from build123d import *
from build123d.topology import SkipClean

# Parameters (mm, degrees)
SALIENTE_EXTRUIR1_DEPTH    = 2.4
CORTAR_EXTRUIR1_DEPTH      = 15.629080627
CORTAR_EXTRUIR1_DEPTH_BACK = 15.629080627
CROQUIS2_R                 = 1.5
CROQUIS3_R                 = 1.5
SALIENTE_EXTRUIR2_DEPTH    = 7.5
CORTAR_EXTRUIR2_DEPTH      = 3.1
REDONDEO1_R                = 2
REDONDEO2_R                = 1


with BuildPart() as part:
    # Croquis1 → Saliente-Extruir1 (new, symmetric)
    with BuildSketch(Plane(origin=(0, 0, 0), x_dir=(0, 0, -1), z_dir=(1, 0, 0))):
        with BuildLine():
            Line((-13, 3.5), (13, 3.5))
            ThreePointArc((13, 3.5), (13.707106781, 3.207106781), (14, 2.5))
            Line((14, 2.5), (14, -2.5))
            Line((14, -2.5), (14, -3.5))
            Line((14, -3.5), (13, -3.5))
            Line((13, -3.5), (-13, -3.5))
            ThreePointArc((-13, -3.5), (-13.707106781, -3.207106781), (-14, -2.5))
            Line((-14, -2.5), (-14, 2.5))
            ThreePointArc((-14, 2.5), (-13.707106781, 3.207106781), (-13, 3.5))
        make_face()
    extrude(amount=SALIENTE_EXTRUIR1_DEPTH, both=True)

    # Croquis2 → Cortar-Extruir1 (cut, two sides: drawn at the far end of the back side and taken through both)
    with BuildSketch(Plane(origin=(0, 0, 0), x_dir=(0, 0, -1), z_dir=(1, 0, 0)).offset(-CORTAR_EXTRUIR1_DEPTH_BACK)):
        with Locations((-10, 0)):
            Circle(CROQUIS2_R)
        with Locations((8, 0)):
            Circle(CROQUIS2_R)
    extrude(amount=CORTAR_EXTRUIR1_DEPTH + CORTAR_EXTRUIR1_DEPTH_BACK, mode=Mode.SUBTRACT)

    # Croquis3 → Saliente-Extruir2 (add, symmetric)
    with SkipClean():  # the faces are left unmerged after this step: merging them gives an invalid solid
        with BuildSketch(Plane(origin=(0, 0, 0), x_dir=(0, 0, -1), z_dir=(1, 0, 0))):
            with BuildLine():
                Line((-14, 2.5), (-14, -2.5))
                ThreePointArc((-14, -2.5), (-13.707106781, -3.207106781), (-13, -3.5))
                Line((-13, -3.5), (0, -3.5))
                Line((0, -3.5), (0, 3.5))
                Line((0, 3.5), (-13, 3.5))
                ThreePointArc((-13, 3.5), (-13.707106781, 3.207106781), (-14, 2.5))
            make_face()
            with Locations((-10, 0)):
                Circle(CROQUIS3_R, mode=Mode.SUBTRACT)
        extrude(amount=SALIENTE_EXTRUIR2_DEPTH, both=True)
    add(part.part.scale(1), mode=Mode.REPLACE)  # the faces are merged on a copy

    # Croquis4 → Cortar-Extruir2 (cut, symmetric)
    with BuildSketch(Plane(origin=(0, 0, 0), x_dir=(0, 0, -1), z_dir=(1, 0, 0))):
        with BuildLine():
            Line((-13, 3.5), (-4, 3.5))
            Line((-4, 3.5), (-4, -3.5))
            Line((-4, -3.5), (-13, -3.5))
            ThreePointArc((-13, -3.5), (-13.707106781, -3.207106781), (-14, -2.5))
            Line((-14, -2.5), (-14, 2.5))
            ThreePointArc((-14, 2.5), (-13.707106781, 3.207106781), (-13, 3.5))
        make_face()
    extrude(amount=CORTAR_EXTRUIR2_DEPTH, both=True, mode=Mode.SUBTRACT)

    # Redondeo1
    redondeo1_edges = [part.edges().sort_by_distance(p)[0] for p in [
        (-2.4, 0, 0),
        (2.4, 0, 0),
        (-7.5, 0, 0),
        (7.5, 0, 0),
    ]]
    fillet(redondeo1_edges, radius=REDONDEO1_R)

    # Redondeo2
    redondeo2_edges = [part.edges().sort_by_distance(p)[0] for p in [
        (3.1, 0, 4),
        (-3.1, 0, 4),
    ]]
    fillet(redondeo2_edges, radius=REDONDEO2_R)


solid = part.part
Work out the finished part from the listing and answer in its coordinate system (mm). A direction names the side the tool comes from. Round coordinates to 2 decimals unless told otherwise and drop trailing zeros. Order: outer loops, then holes, each group sorted by start corner. A loop starts at its lowest first (then second) coordinate and runs counter-clockwise, first axis right, second up. Notation, with made-up numbers: M 51.25,-25.75 L 109.25,-25.75 A23 cw 109.25,-9.75 Z; hole C 21,10.25 d4. An arc over 180 degrees is marked long. Put each result on its own line as item: value. Start each with the question number.
Q1. A tool of negligible diameter and unlimited length cuts with its end or side. For faces 1 (the cylindrical face through (-2.815, -0.049, 4.301)), 2 (the flat face through (-2.4, -2, -8)), 3 (the cylindrical face through (-5.269, -3.199, 13.715)), 4 (the flat face through (5, 0, 0)), from which of +Z, -Z, +X, -X, +Y, -Y can it reach the whole face along a straight path? Write none if from no direction.
Q2. Section C-C, the plane x = 0.75 is taken. Write down the section's boundary in (y, z).
Q3. Section B-B, the plane y = 0 is taken. Give the number of separate pieces and of enclosed holes in the cut face, and give its area (3 significant figures).
Q4. Straight lines are drawn through the part: L1, parallel to Z at x = -0.8, y = 0; L2, parallel to Y at x = 4.7, z = 10; L3, parallel to X at y = -3, z = 8.5. For each, find the intervals that lie inside material, in ascending order. Write a range as [from, to].
Q5. Section A-A, the plane z = 10 is taken. Write down the section's boundary in (x, y), and give its area (3 significant figures).
Q6. Flat-ended cylindrical pins translate along their axes: pin 1 (3 mm diameter, centred on x = 1, y = 0, fed in from +Z); pin 2 (4 mm diameter, centred on y = 1, z = -7.5, fed in from +X); pin 3 (3.5 mm diameter, centred on x = 1, y = 0.5, fed in from +Z). Find the tip coordinate at first contact, or state that the pin passes through.
Q7. Section D-D, the plane z = -8 is taken. Write down the section's boundary in (x, y).
Q8. For a pull along Y with two mould halves and no side action, classify faces 5 (the flat face through (-5, 0, 14)), 6 (the flat face through (0, -3.5, 3)), 7 (the cylindrical face through (-5.269, 3.215, 13.699)), 8 (the cylindrical face through (-5.27, 0.07, 11.5)) as pulls with the +Y half, pulls with the -Y half, needs draft (parallel to the pull), parting line crosses it, or undercut.
Findings below:
1. face 1: +Z, +Y, -Y
1. face 2: -Z, -X, +Y, -Y
1. face 3: +Z, +X, -X, -Y
1. face 4: -Z, +X, +Y, -Y
2. outline: M -3.5,-14 L 2.5,-14 A1 ccw 3.5,-13 L 3.5,4 L -3.5,4 Z; hole C 0,-8 d3
3. separate pieces: 4
3. enclosed holes: 0
3. area: 175 mm^2
4. L1: z = [-14, -9.5], [-6.5, 4]
4. L2: y = [-3.5, -1.5], [1.5, 3.5]
4. L3: x = [-7.5, -3.1], [3.1, 7.5]
5. outline: M -7.5,-3.5 L -3.1,-3.5 L -3.1,-1.5 L -7.5,-1.5 Z; M -7.5,1.5 L -3.1,1.5 L -3.1,3.5 L -7.5,3.5 Z; M 3.1,-3.5 L 7.5,-3.5 L 7.5,-1.5 L 3.1,-1.5 Z; M 3.1,1.5 L 7.5,1.5 L 7.5,3.5 L 3.1,3.5 Z
5. area: 35.2 mm^2
6. pin 1: stops at z = 4.08
6. pin 2: stops at x = 2.4
6. pin 3: stops at z = 4.24
7. outline: M -2.4,-3.5 L 2.4,-3.5 L 2.4,-1.5 L -2.4,-1.5 Z; M -2.4,1.5 L 2.4,1.5 L 2.4,3.5 L -2.4,3.5 Z
8. face 5: needs draft
8. face 6: pulls with the -Y half
8. face 7: pulls with the +Y half
8. face 8: undercut
